Work out the finished part from the listing and answer in its coordinate system (mm). Face numbers are marked on the shaded views. Round coordinates to 2 decimals unless told otherwise and drop trailing zeros. Loops run counter-clockwise (first coordinate to the right, second up) from the corner with the lowest first, then second, coordinate; pieces in that order, holes last. Notation, with made-up numbers: (3, 88.25) -> (34, 88.25) arc R31 ccw to (34, 125.25) -> close; hole circle Ø7 at (57.5, -16.75). An arc over 180 degrees is marked (long way). Use one line per item in the form item = value.
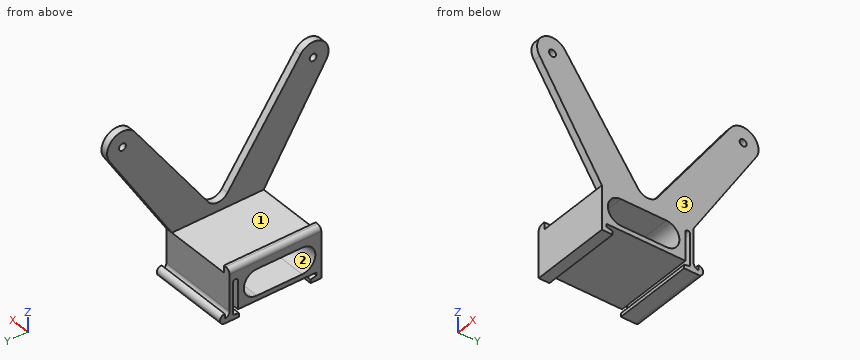
```python
from build123d import *

# Parameters (mm, degrees)
SKETCH001_R  = 1.45
PAD_DEPTH    = 33.9
SKETCH002_W  = 200
SKETCH002_H  = 80
POCKET_DEPTH = 30.9
SKETCH003_W  = 38.5
SKETCH003_H  = 3
PAD001_DEPTH = 3
FILLET_R     = 2
FILLET001_R  = 5


with BuildPart() as part:
    # Sketch001 → Pad (new body)
    with BuildSketch(Plane.YZ):
        with BuildLine():
            Line((-15, -3.3), (-19.5, -3.3))
            Line((-19.5, -3.3), (-19.5, 15))
            Line((-19.5, 15), (-45.596074, 56.3914))
            ThreePointArc((-34.903926, 63.6086), (-43.8586, 65.346074), (-45.596074, 56.3914))
            Line((-34.903926, 63.6086), (-0.25, 15))
            Line((-0.25, 15), (34.403926, 63.6086))
            ThreePointArc((45.096074, 56.3914), (43.3586, 65.346074), (34.403926, 63.6086))
            Line((45.096074, 56.3914), (19, 15))
            Line((19, 15), (19, 0.7))
            ThreePointArc((19, 0.7), (19.585786, -0.714214), (21, -1.3))
            Line((21, -1.3), (21, 0.7))
            ThreePointArc((21, -3.3), (23, -1.3), (21, 0.7))
            Line((21, -3.3), (15, -3.3))
            Line((15, -3.3), (15, -1.8))
            Line((15, -1.8), (17.5, -1.3))
            Line((17.5, -1.3), (17.5, 0))
            Line((17.5, 12), (17.5, 0))
            ThreePointArc((17.5, 12), (16.5, 13), (15.5, 12))
            Line((15.5, 0), (15.5, 12))
            Line((-17.5, 0), (15.5, 0))
            Line((-17.5, 0), (-17.5, -1.3))
            Line((-17.5, -1.3), (-15, -1.8))
            Line((-15, -1.8), (-15, -3.3))
        make_face()
        with Locations((-40.25, 60)):
            Circle(SKETCH001_R, mode=Mode.SUBTRACT)
        with Locations((39.75, 60)):
            Circle(SKETCH001_R, mode=Mode.SUBTRACT)
        with BuildLine():
            ThreePointArc((-11.5, 13), (-17, 7.5), (-11.5, 2))
            Line((-11.5, 2), (7.5, 2))
            ThreePointArc((7.5, 2), (13, 7.5), (7.5, 13))
            Line((-11.5, 13), (7.5, 13))
        make_face(mode=Mode.SUBTRACT)
    extrude(amount=PAD_DEPTH)

    # Sketch002 (on Face30 of Pad) → Pocket (cut)
    with BuildSketch(Plane(origin=(0, 0, 0), x_dir=(0, 1, 0), z_dir=(-1, 0, 0))):
        with Locations((19, -55)):
            Rectangle(SKETCH002_W, SKETCH002_H)
    extrude(amount=-POCKET_DEPTH, mode=Mode.SUBTRACT)

    # Sketch003 (on Face18 of Pocket) → Pad001 (join)
    with BuildSketch(Plane(origin=(0, 0, 15), x_dir=(0, -1, 0), z_dir=(0, 0, 1))):
        with Locations((0.25, 1.5)):
            Rectangle(SKETCH003_W, SKETCH003_H)
    extrude(amount=PAD001_DEPTH)

    # Fillet
    fillet_edges = [part.edges().sort_by_distance(p)[0] for p in [
        (0, -0.25, 18),
    ]]
    fillet(fillet_edges, radius=FILLET_R)

    # Fillet001
    fillet001_edges = [part.edges().sort_by_distance(p)[0] for p in [
        (32.4, -0.25, 15),
    ]]
    fillet(fillet001_edges, radius=FILLET001_R)


solid = part.part
```
(1) Find section A-A, the plane z = 4.5. Write down the section's boundary in (x, y), then the cut area to 3 significant figures.
Completed:
outline = (0, -19.5) -> (33.9, -19.5) -> (33.9, -16.11) -> (0, -16.11) -> close; (0, 12.11) -> (33.9, 12.11) -> (33.9, 15.5) -> (0, 15.5) -> close; (0, 17.5) -> (33.9, 17.5) -> (33.9, 19) -> (0, 19) -> close
area = 281 mm2
(2) Consider L1, parallel to Y at x = 31.8, z = 60; L2, parallel to Y at x = 31, z = 8.5; L3, parallel to Z at x = 3.5, y = -3. Determine where each line is inside the solid, lowest interval first.
Completed:
L1 = -46.7 to -41.7, -38.8 to -32.33, 31.83 to 38.3, 41.2 to 46.2
L2 = -19.5 to -16.91, 12.91 to 15.5, 17.5 to 19
L3 = 0 to 2, 13 to 15
(3) Find section C-C, the plane y = 39.75. Write down the section's boundary in (x, z).
Completed:
outline = (30.9, 47.91) -> (33.9, 47.91) -> (33.9, 58.55) -> (30.9, 58.55) -> close; (30.9, 61.45) -> (33.9, 61.45) -> (33.9, 66.45) -> (30.9, 66.45) -> close
(4) Find section B-B, the plane x = 28. Write down the section's boundary in (y, z), then the cut area to 3 significant figures.
Completed:
outline = (-19.5, -3.3) -> (-15, -3.3) -> (-15, -1.8) -> (-17.5, -1.3) -> (-17.5, 0) -> (15.5, 0) -> (15.5, 12) arc R1 cw to (17.5, 12) -> (17.5, -1.3) -> (15, -1.8) -> (15, -3.3) -> (21, -3.3) arc R2 ccw to (21, 0.7) -> (21, -1.3) arc R2 cw to (19, 0.7) -> (19, 15) -> (-19.5, 15) -> close; hole (-11.5, 2) -> (7.5, 2) arc R5.5 ccw to (7.5, 13) -> (-11.5, 13) arc R5.5 ccw to start
area = 279 mm2
(5) Find section D-D, the plane z = 44.5. Write down the section's boundary in (x, y), then the cut area to 3 significant figures.
Completed:
outline = (30.9, -38.1) -> (33.9, -38.1) -> (33.9, -21.28) -> (30.9, -21.28) -> close; (30.9, 20.78) -> (33.9, 20.78) -> (33.9, 37.6) -> (30.9, 37.6) -> close
area = 101 mm2
(6) Given P1, Ø1.1, axis at x = 2.5, y = -4, coming from the +Z side; P2, Ø3.5, axis at y = -40.25, z = 60, coming from the +X side; P3, Ø3, axis at y = -35.5, z = 49, coming from the -X side; P4, Ø2.5, axis at y = 39.75, z = 60, coming from the -X side, each flat-ended and moving along its own axis, determine where each tip first touches the part or whether it passes through.
Completed:
P1 = 18
P2 = 33.9
P3 = 30.9
P4 = through
(7) For a pull along Z with two mould halves and no side action, classify the marked faces 1, 2 and 3 as +Z half, -Z half, draft (parallel to the pull), parting line (faces both ways), or undercut.
Completed:
face_1 = +Z half
face_2 = undercut
face_3 = draft
